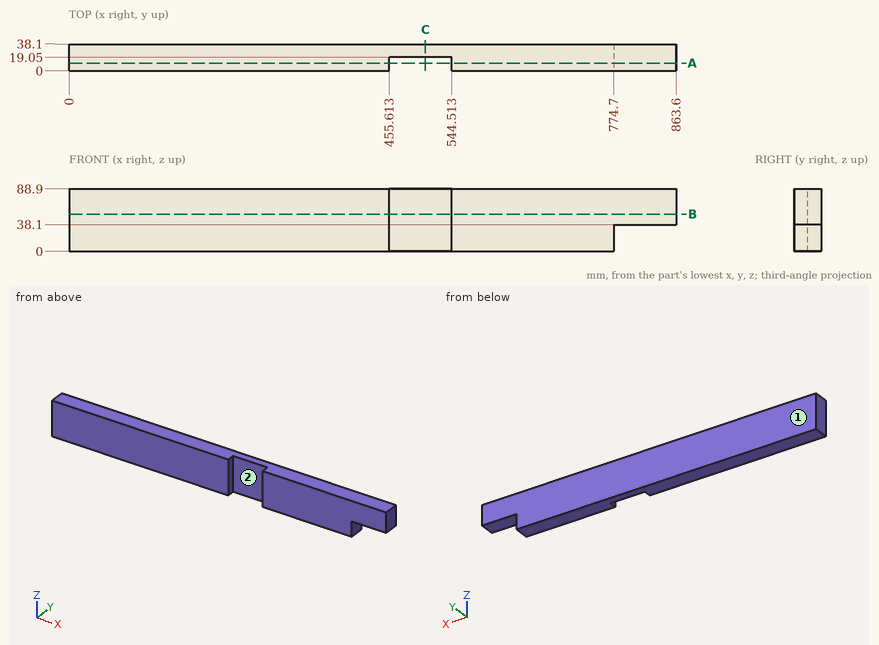
Study the drawing (mm; zero at the part's minimum x, y, z) and answer. Coordinates: 2 decimals unless noted, no trailing zeros. Loops run counter-clockwise (first coordinate to the right, second up) from the corner with the lowest first, then second, coordinate; pieces in that order, holes last. Notation, with made-up numbers: (40, 55.25) -> (47, 55.25) arc R19 cw to (47, 63.25) -> close; hole circle Ø3 at (36.25, 79). An arc over 180 degrees is marked (long way). Answer as CSV lines item,"result".
1) Straight lines are drawn through the part: probe 1 along X at (y, z) = (10, 54.5); probe 2 along X at (y, z) = (12, 16.5); probe 3 along X at (y, z) = (27.5, 32). For each, find the intervals that lie inside material, in ascending order.
A:
probe 1,"x = 0 to 455.61, 544.51 to 863.6"
probe 2,"x = 0 to 455.61, 544.51 to 774.7"
probe 3,"x = 0 to 774.7"
2) Flat-ended cylindrical pins translate along their axes: pin 1 (2 mm diameter, centred on y = 17.5, z = 20, fed in from +X); pin 2 (1 mm diameter, centred on y = 26.5, z = 45.5, fed in from -X). Find the tip coordinate at first contact, or state that the pin passes through.
A:
pin 1,"stops at x = 774.7"
pin 2,"stops at x = 0"
3) For a pull along X with two mould halves and no side action, classify the marked faces 1 and 2 as released by +X, released by -X, zero draft, split by the parting line, or undercut.
A:
face 1,"zero draft"
face 2,"undercut"
4) The part is cut by section C-C (x = 507). Give the vertices of the cut face in (y, z), and give its area (3 significant figures).
A:
outline,"(19.05, 0) -> (38.1, 0) -> (38.1, 88.9) -> (19.05, 88.9) -> close"
area,"1,690 mm²"
5) The part is cut by section B-B (z = 53). Give the vertices of the cut face in (x, y), and give its area (3 significant figures).
A:
outline,"(0, 0) -> (455.61, 0) -> (455.61, 19.05) -> (544.51, 19.05) -> (544.51, 0) -> (863.6, 0) -> (863.6, 38.1) -> (0, 38.1) -> close"
area,"31,200 mm²"
6) The part is cut by section A-A (y = 11). Give the vertices of the cut face in (x, z).
A:
outline,"(0, 0) -> (455.61, 0) -> (455.61, 88.9) -> (0, 88.9) -> close; (544.51, 0) -> (774.7, 0) -> (774.7, 38.1) -> (863.6, 38.1) -> (863.6, 88.9) -> (544.51, 88.9) -> close"
